from build123d import *

# Parameters (mm, degrees)
F0_W     = 100
F0_H     = 100
F1_DEPTH = 100
F2_W     = 100
F2_H     = 80
F3_DEPTH = 40
F4_W     = 60
F4_H     = 40
F5_DEPTH = 2000


with BuildPart() as f1:
    # F0 (on Top) → F1 (new body)
    with BuildSketch(Plane.XY):
        Rectangle(F0_W, F0_H)
    extrude(amount=F1_DEPTH)

    # F2 (on face) → F3 (cut)
    with BuildSketch(Plane.XY.offset(100)):
        with Locations((0, -10)):
            Rectangle(F2_W, F2_H)
    extrude(amount=-F3_DEPTH, mode=Mode.SUBTRACT)

    # F4 (on face) → F5 (cut)
    with BuildSketch(Plane.XZ.offset(50)):
        with Locations((0, 20)):
            Rectangle(F4_W, F4_H)
    extrude(amount=-F5_DEPTH, mode=Mode.SUBTRACT)


solid = f1.part
Read the model definition and answer for the solid it produces. Units are mm, in the model's axes. A direction names the side the tool comes from. Give positions to 0.01 mm unless a question says otherwise; leave off trailing zeros. Write each loop counter-clockwise with the first axis right and the second up, starting at its lowest first coordinate (ties: lowest second). Pieces come first, ordered by that corner, then holes. Notation, with made-up numbers: (10, 70.25) - (43, 70.25) arc R25 cw to (43, 88.25) - close; hole circle Ø10 at (32.5, -20.75). An arc over 180 degrees is marked (long way). Use CSV: the item, a comma, the result in double quotes. Start each with the question number.
(1) Given P1, Ø2, axis at x = 13, y = 26.5, coming from the -Z side; P2, Ø4, axis at x = -18, z = 75.5, coming from the -Y side; P3, Ø4, axis at x = 31, y = -16, coming from the -Z side; P4, Ø6, axis at x = 33.5, y = -12, coming from the +Z side, each flat-ended and moving along its own axis, determine where each tip first touches the part or whether it passes through.
(2) Consider line 1 along X through (y, z) = (20, 18.5); line 2 along Y through (x, z) = (8, 83.5); line 3 along Z through (x, y) = (6, -44). Determine where each line is inside the solid, lowest interval first.
(3) Find section D-D (z = 71.5). Give the vertices of the cut face in (x, y).
(4) For faces 5 (the flat face through (-1, 30, 80)), 6 (the flat face through (-30, -1, 20)), 7 (the flat face through (-1, 40, 100)), determine the directions among +Z, -Z, +X, -X, +Y, -Y from which every point of the face is accessible in a straight line to the end or side of a thin tool.
(5) Find section B-B (y = 32). Give the vertices of the cut face in (x, z).
(6) Find section A-A (z = 7). Give the vertices of the cut face in (x, y), plus the area to 3 significant figures.
(7) Find section C-C (x = 39.5). Give the vertices of the cut face in (y, z), plus the area to 3 significant figures.
(8) Determine the mould class of faces 1 (the flat face through (30, -1, 20)), 2 (the flat face through (50, 10, 38)), 3 (the flat face through (-1, -9, 60)), 4 (the flat face through (0, -1, 40)) for opening direction X: +X half, -X half, draft (parallel to the pull), parting line (faces both ways), or undercut.
Findings below:
1,P1,"z = 40"
1,P2,"y = 30"
1,P3,"z = 0"
1,P4,"z = 60"
2,line 1,"-50 to -30, 30 to 50"
2,line 2,"30 to 50"
2,line 3,"40 to 60"
3,outline,"(-50, 30) - (50, 30) - (50, 50) - (-50, 50) - close"
4,face 5,"+Z, +X, -X, -Y"
4,face 6,"-Z, +Y, -Y"
4,face 7,"+Z, +X, -X, +Y, -Y"
5,outline,"(-50, 0) - (-30, 0) - (-30, 40) - (30, 40) - (30, 0) - (50, 0) - (50, 100) - (-50, 100) - close"
6,outline,"(-50, -50) - (-30, -50) - (-30, 50) - (-50, 50) - close; (30, -50) - (50, -50) - (50, 50) - (30, 50) - close"
6,area,"4,000 mm2"
7,outline,"(-50, 0) - (50, 0) - (50, 100) - (30, 100) - (30, 60) - (-50, 60) - close"
7,area,"6,800 mm2"
8,face 1,"undercut"
8,face 2,"+X half"
8,face 3,"draft"
8,face 4,"undercut"
